from build123d import *

# Parameters (mm, degrees)
SKETCH1_W             = 575
SKETCH1_H             = 385
BOSS_EXTRUDE1_DEPTH   = 50
CAVITY2_START         = -50
CAVITY2_OUTLINE_R     = 10
CAVITY2_DEPTH         = 100
CAVITY2_2_OUTLINE_R   = 15.25
CAVITY2_2_OUTLINE_R_2 = 10.25
CAVITY2_2_DEPTH       = 20


# Read off the part's stored shape, not the designer's step: Cavity2
with BuildPart() as part:
    # Sketch1 → Boss-Extrude1 (new, symmetric)
    with BuildSketch(Plane(origin=(0, 0, 0), x_dir=(1, 0, 0), z_dir=(0, 1, 0))):
        Rectangle(SKETCH1_W, SKETCH1_H)
    extrude(amount=BOSS_EXTRUDE1_DEPTH, both=True)

    # Cavity2 outline → Cavity2 (cut)
    with BuildSketch(Plane(origin=(0, 0, 0), x_dir=(1, 0, 0), z_dir=(0, 1, 0)).offset(CAVITY2_START)):
        Circle(CAVITY2_OUTLINE_R)
    extrude(amount=CAVITY2_DEPTH, mode=Mode.SUBTRACT)

    # Cavity2 2 outline → Cavity2 2 (cut)
    with BuildSketch(Plane(origin=(0, 0, 0), x_dir=(1, 0, 0), z_dir=(0, 1, 0)).offset(CAVITY2_START)):
        Circle(CAVITY2_2_OUTLINE_R)
        Circle(CAVITY2_2_OUTLINE_R_2, mode=Mode.SUBTRACT)
    extrude(amount=CAVITY2_2_DEPTH, mode=Mode.SUBTRACT)


solid = part.part
The model under review builds one solid part; all positions refer to its coordinate system, in mm. A direction names the side the tool comes from. Coordinates: 2 decimals unless noted, no trailing zeros. Write each loop counter-clockwise with the first axis right and the second up, starting at its lowest first coordinate (ties: lowest second). Pieces come first, ordered by that corner, then holes. Notation, with made-up numbers: (14.25, 4.5) - (47.25, 4.5) arc R26 cw to (47.25, 37.5) - close; hole circle Ø8 at (7, 48.25). An arc over 180 degrees is marked (long way). Answer as a JSON object with one key per item and string values. Group by question number.
1. To check wall thickness, follow probe 1 along X at (y, z) = (-36.5, 0); probe 2 along Z at (x, y) = (0, 5); probe 3 along X at (y, z) = (-5, -7.5). State the ranges of each line that lie inside material, in increasing order.
2. Add section B-B (x = 0). Give the boundary of the cut face in (y, z), plus the area to 3 significant figures.
3. Mouldability with a two-part tool opening along X and no side actions: class faces 1 (the face through (287.5, 1, 3)), 2 (the face through (-2.222, -40.14, 10.006)), 3 (the face through (-4, 1, -192.5)), 4 (the face through (-287.5, 1, 3)) as pulls with the +X half, pulls with the -X half, needs draft (parallel to the pull), parting line crosses it, or undercut.
4. Machinability: for faces 5 (the face through (-12.1, -40.14, 9.28)), 6 (the face through (-2.17, -0.7, 9.76)), which of the approach directions +Z, -Z, +X, -X, +Y, -Y give a long, thin tool a straight path to every point of the face, cutting with its end or side? Answer none if there is none.
5. Add section A-A (z = 0). Give the boundary of the cut face in (x, y).
Findings:
{
 "1": {"probe 1": "-287.5 to -15.25, -10.25 to -10, 10 to 10.25, 15.25 to 287.5", "probe 2": "-192.5 to -10, 10 to 192.5", "probe 3": "-287.5 to -6.61, 6.61 to 287.5"},
 "2": {"outline": "(-50, -192.5) - (50, -192.5) - (50, -10) - (-50, -10) - (-50, -10.25) - (-30, -10.25) - (-30, -15.25) - (-50, -15.25) - close; (-50, 10) - (50, 10) - (50, 192.5) - (-50, 192.5) - (-50, 15.25) - (-30, 15.25) - (-30, 10.25) - (-50, 10.25) - close", "area": "36,300 mm²"},
 "3": {"face 1": "pulls with the +X half", "face 2": "undercut", "face 3": "needs draft", "face 4": "pulls with the -X half"},
 "4": {"face 5": "-Y", "face 6": "+Y, -Y"},
 "5": {"outline": "(-287.5, -50) - (-15.25, -50) - (-15.25, -30) - (-10.25, -30) - (-10.25, -50) - (-10, -50) - (-10, 50) - (-287.5, 50) - close; (10, -50) - (10.25, -50) - (10.25, -30) - (15.25, -30) - (15.25, -50) - (287.5, -50) - (287.5, 50) - (10, 50) - close"}
}
